Source: three-view drawing plus pictorial views. Frame: mm from the lowest corner of the part. A direction names the side the tool comes from. Give positions to 0.01 mm unless a question says otherwise; leave off trailing zeros. Order: outer loops, then holes, each group sorted by start corner. A loop starts at its lowest first (then second) coordinate and runs counter-clockwise, first axis right, second up. Notation, with made-up numbers: (1.25, 64) - (9.25, 64) arc R27 cw to (9.25, 81) - close; hole circle Ø5 at (-26.75, 60.25). An arc over 180 degrees is marked (long way). Use CSV: the item, a comma, the result in double quotes.
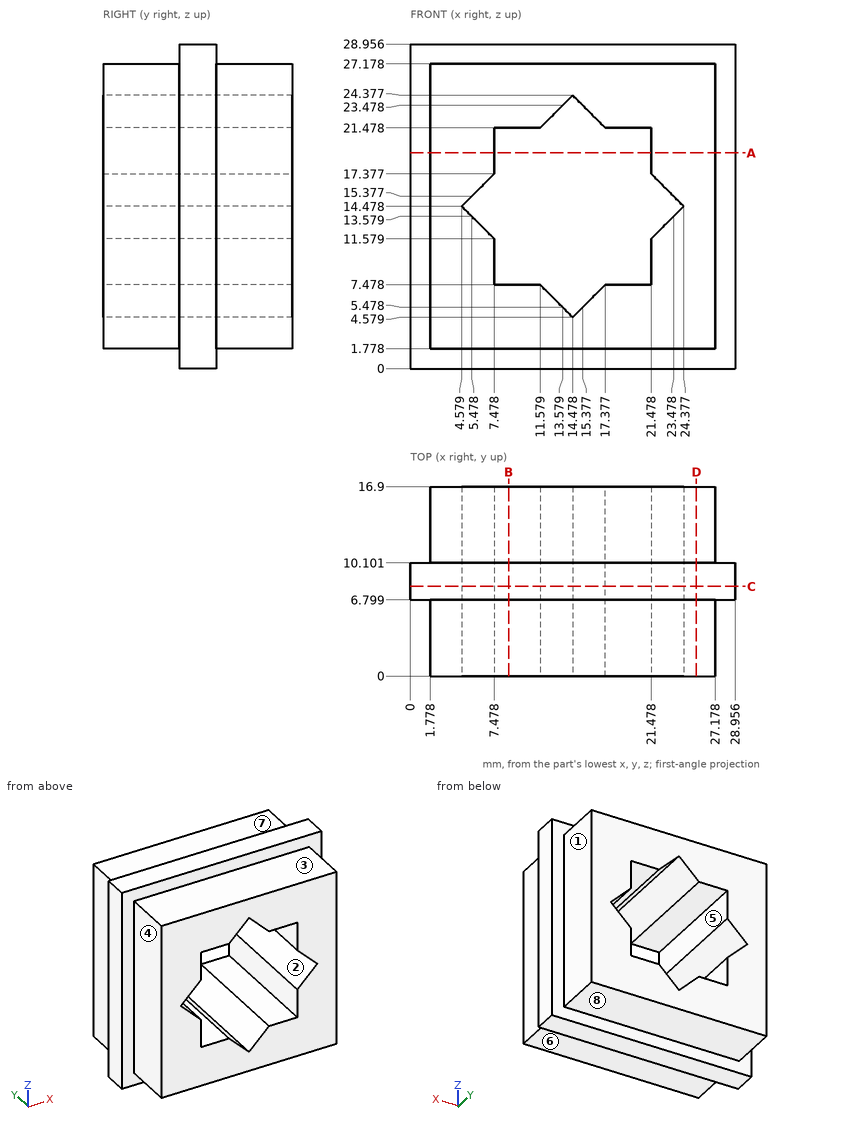
Item 1: Set-up query: the marked faces 4, 5, 6, 7 and 8. Return all of +Z, -Z, +X, -X, +Y, -Y with unobstructed straight access to the full face (end or side cutting, diameter ignored); none if empty.
Filled in:
face 4,"+Z, -Z, -X, -Y"
face 5,"+Y, -Y"
face 6,"-Z, +X, -X, -Y"
face 7,"+Z, +X, -X, +Y"
face 8,"-Z, +X, -X, +Y"
Item 2: First-contact query: pin 1 (4 mm diameter, centred on x = 20, y = 5.5, fed in from -Z); pin 2 (3.5 mm diameter, centred on y = 13, z = 14, fed in from +X); pin 3 (2 mm diameter, centred on y = 4, z = 8.5, fed in from -X); pin 4 (4 mm diameter, centred on x = 15, y = 13.5, fed in from -Z). Flat tips, straight axial feed; report the tip coordinate or a pass-through.
Filled in:
pin 1,"stops at z = 0"
pin 2,"stops at x = 27.18"
pin 3,"stops at x = 1.78"
pin 4,"stops at z = 1.78"
Item 3: Section A-A on z = 19.25. Return the cut outline in (x, y).
Filled in:
outline,"(0, 6.8) - (1.78, 6.8) - (1.78, 0) - (7.48, 0) - (7.48, 16.9) - (1.78, 16.9) - (1.78, 10.1) - (0, 10.1) - close; (21.48, 0) - (27.18, 0) - (27.18, 6.8) - (28.96, 6.8) - (28.96, 10.1) - (27.18, 10.1) - (27.18, 16.9) - (21.48, 16.9) - close"
Item 4: Mould query, pull axis X, two halves, no side actions, for the marked faces 1, 2 and 3. Classes: released by +X, released by -X, zero draft, split by the parting line, or undercut.
Filled in:
face 1,"released by +X"
face 2,"undercut"
face 3,"zero draft"
Item 5: Section B-B on x = 8.75. Return the cut outline in (y, z).
Filled in:
outline,"(0, 1.78) - (6.8, 1.78) - (6.8, 0) - (10.1, 0) - (10.1, 1.78) - (16.9, 1.78) - (16.9, 7.48) - (0, 7.48) - close; (0, 21.48) - (16.9, 21.48) - (16.9, 27.18) - (10.1, 27.18) - (10.1, 28.96) - (6.8, 28.96) - (6.8, 27.18) - (0, 27.18) - close"
Item 6: Material intervals for line 1 (Z direction, x = 19, y = 11); line 2 (X direction, y = 2.5, z = 25.75), sorted ascending. Write a range as from..to.
Filled in:
line 1,"z = 1.78..7.48, 21.48..27.18"
line 2,"x = 1.78..27.18"
Item 7: Section C-C on y = 8. Return the cut outline in (x, z), then the cut area to 3 significant figures.
Filled in:
outline,"(0, 0) - (28.96, 0) - (28.96, 28.96) - (0, 28.96) - close; hole (4.58, 14.48) - (7.48, 11.58) - (7.48, 7.48) - (11.58, 7.48) - (14.48, 4.58) - (17.38, 7.48) - (21.48, 7.48) - (21.48, 11.58) - (24.38, 14.48) - (21.48, 17.38) - (21.48, 21.48) - (17.38, 21.48) - (14.48, 24.38) - (11.58, 21.48) - (7.48, 21.48) - (7.48, 17.38) - close"
area,"609 mm2"
Item 8: Section D-D on x = 25.5. Return the cut outline in (y, z).
Filled in:
outline,"(0, 1.78) - (6.8, 1.78) - (6.8, 0) - (10.1, 0) - (10.1, 1.78) - (16.9, 1.78) - (16.9, 27.18) - (10.1, 27.18) - (10.1, 28.96) - (6.8, 28.96) - (6.8, 27.18) - (0, 27.18) - close"
